```python
from build123d import *

# Parameters (mm, degrees)
SKETCH1_W           = 350
SKETCH1_H           = 350
BOSS_EXTRUDE1_DEPTH = 3
SKETCH3_W           = 18
SKETCH3_H           = 100
CUT_EXTRUDE1_DEPTH  = 3
SKETCH4_W           = 56
SKETCH4_H           = 70
CUT_EXTRUDE2_DEPTH  = 3
SKETCH5_R           = 2.5
SKETCH5_R_2         = 1.6
CUT_EXTRUDE3_DEPTH  = 3


with BuildPart() as part:
    # Sketch1 → Boss-Extrude1 (new body)
    with BuildSketch(Plane(origin=(0, 0, 0), x_dir=(1, 0, 0), z_dir=(0, 1, 0))):
        Rectangle(SKETCH1_W, SKETCH1_H)
    extrude(amount=BOSS_EXTRUDE1_DEPTH)

    # Sketch3 → Cut-Extrude1 (cut)
    with BuildSketch(Plane(origin=(0, 3, 0), x_dir=(1, 0, 0), z_dir=(0, 1, 0))):
        with Locations((-140, 0)):
            Rectangle(SKETCH3_W, SKETCH3_H)
        with Locations((140, 0)):
            Rectangle(SKETCH3_W, SKETCH3_H)
    extrude(amount=-CUT_EXTRUDE1_DEPTH, mode=Mode.SUBTRACT)

    # Sketch4 → Cut-Extrude2 (cut)
    with BuildSketch(Plane(origin=(0, 3, 0), x_dir=(1, 0, 0), z_dir=(0, 1, 0))):
        with Locations((0, 135.000000303)):
            Rectangle(SKETCH4_W, SKETCH4_H)
        with Locations((0, -135.000003084)):
            Rectangle(SKETCH4_W, SKETCH4_H)
    extrude(amount=-CUT_EXTRUDE2_DEPTH, mode=Mode.SUBTRACT)

    # Sketch5 → Cut-Extrude3 (cut)
    with BuildSketch(Plane(origin=(0, 3, 0), x_dir=(1, 0, 0), z_dir=(0, 1, 0))):
        with Locations((-158, 21)):
            Circle(SKETCH5_R)
        with Locations((-158, -21)):
            Circle(SKETCH5_R)
        with Locations((-122, 21)):
            Circle(SKETCH5_R)
        with Locations((-122, -21)):
            Circle(SKETCH5_R)
        with Locations((158, 21)):
            Circle(SKETCH5_R)
        with Locations((158, -21)):
            Circle(SKETCH5_R)
        with Locations((122, 21)):
            Circle(SKETCH5_R)
        with Locations((122, -21)):
            Circle(SKETCH5_R)
        with Locations((-39.999996759, -135.000003084)):
            Circle(SKETCH5_R)
        with Locations((39.999996759, -135.000003084)):
            Circle(SKETCH5_R)
        with Locations((-39.999996759, 135.000000303)):
            Circle(SKETCH5_R)
        with Locations((39.999996759, 135.000000303)):
            Circle(SKETCH5_R)
        with Locations((-150, 150)):
            Circle(SKETCH5_R_2)
        with Locations((150, 150)):
            Circle(SKETCH5_R_2)
        with Locations((150, -150)):
            Circle(SKETCH5_R_2)
        with Locations((-150, -150)):
            Circle(SKETCH5_R_2)
    extrude(amount=-CUT_EXTRUDE3_DEPTH, mode=Mode.SUBTRACT)


solid = part.part
```
Can you work these out from the model? Positions are in its coordinate system, mm. Round coordinates to 2 decimals unless told otherwise and drop trailing zeros. Loops run counter-clockwise (first coordinate to the right, second up) from the corner with the lowest first, then second, coordinate; pieces in that order, holes last.
Item 1: Suppose I cut it at C-C, the plane y = 2.45. State how many separate pieces and enclosed holes the cut face has, then the cut area to 3 significant figures.
Item 2: Will this pin go through, and if not, where does the flat tip stop? pin 1 Ø6.5 at (x, z) = (158, -21) entering from +Y.
Item 3: Please list where these lines run through material, in increasing order: L1, parallel to X at y = 2.6, z = 134.5; L2, parallel to X at y = 1.7, z = -135; L3, parallel to Z at x = 16.5, y = 1.8.
Item 4: Suppose I cut it at B-B, the plane z = 28. Write out the boundary of the cut face in (x, y), then the cut area to 3 significant figures.
Item 5: Suppose I cut it at A-A, the plane z = -112.5. Write out the boundary of the cut face in (x, y), then the cut area to 3 significant figures.
Reported:
1. separate pieces: 1
1. enclosed holes: 20
1. area: 111,000 mm2
2. pin 1: stops at y = 3
3. L1: x = -175 to -42.45, -37.55 to -28, 28 to 37.55, 42.45 to 175
3. L2: x = -175 to -42.5, -37.5 to -28, 28 to 37.5, 42.5 to 175
3. L3: z = -175 to -170, -100 to 100, 170 to 175
4. outline: (-175, 0) - (-149, 0) - (-149, 3) - (-175, 3) - close; (-131, 0) - (131, 0) - (131, 3) - (-131, 3) - close; (149, 0) - (175, 0) - (175, 3) - (149, 3) - close
4. area: 942 mm2
5. outline: (-175, 0) - (-28, 0) - (-28, 3) - (-175, 3) - close; (28, 0) - (175, 0) - (175, 3) - (28, 3) - close
5. area: 882 mm2
